Here's how the part is built. I have some questions about the finished solid (model axes, mm). A direction names the side the tool comes from. Coordinates: 2 decimals unless noted, no trailing zeros. Write each loop counter-clockwise with the first axis right and the second up, starting at its lowest first coordinate (ties: lowest second). Pieces come first, ordered by that corner, then holes.
from build123d import *

# Parameters (mm, degrees)
F0_W      = 80
F0_H      = 60
F1_DEPTH  = 10
F2_R      = 13.15
F3_DEPTH  = 10.001
F4_R      = 4
F5_DEPTH  = 10.001
F6_R      = 5
F7_W      = 14
F7_H      = 22
F8_DEPTH  = 5
F9_R      = 5
F10_R     = 13.15
F10_R_2   = 11.15
F11_DEPTH = 2.4


with BuildPart() as f1:
    # F0 (on Front) → F1 (new body)
    with BuildSketch(Plane.XZ):
        with Locations((0, 10)):
            Rectangle(F0_W, F0_H)
    extrude(amount=F1_DEPTH)

    # F2 (on face) → F3 (cut, through all)
    with BuildSketch(Plane.XZ.offset(10)):
        with Locations((0, 10)):
            Circle(F2_R)
    extrude(amount=-F3_DEPTH, mode=Mode.SUBTRACT)

    # F4 (on face) → F5 (cut, through all)
    with BuildSketch(Plane.XZ.offset(10)):
        with Locations((-31, 31)):
            Circle(F4_R)
        with Locations((31, 31)):
            Circle(F4_R)
        with Locations((-31, -11)):
            Circle(F4_R)
        with Locations((31, -11)):
            Circle(F4_R)
    extrude(amount=-F5_DEPTH, mode=Mode.SUBTRACT)

    # F6
    f6_edges = [f1.edges().sort_by_distance(p)[0] for p in [
        (40, -5, 40),
        (40, -5, -20),
        (-40, -5, -20),
        (-40, -5, 40),
    ]]
    fillet(f6_edges, radius=F6_R)

    # F7 (on face) → F8 (cut)
    with BuildSketch(Plane.XZ.offset(10)):
        Polygon((-24.5, 34.7527767497), (-31, 38.5055534995), (-37.5, 34.7527767497), (-37.5, 27.2472232503), (-31, 23.4944465005), (-24.5, 27.2472232503), align=None)
        Polygon((24.5, 34.7527767497), (24.5, 27.2472232503), (31, 23.4944465005), (37.5, 27.2472232503), (37.5, 34.7527767497), (31, 38.5055534995), align=None)
        Polygon((24.5, -7.2472232503), (24.5, -14.7527767497), (31, -18.5055534995), (37.5, -14.7527767497), (37.5, -7.2472232503), (31, -3.4944465005), align=None)
        Polygon((-24.5, -7.2472232503), (-31, -3.4944465005), (-37.5, -7.2472232503), (-37.5, -14.7527767497), (-31, -18.5055534995), (-24.5, -14.7527767497), align=None)
        with BuildLine():
            ThreePointArc((13.6106575888, 21), (16.499037969, 15.8336734651), (17.5, 10))
            ThreePointArc((17.5, 10), (16.499037969, 4.1663265349), (13.6106575888, -1))
            Line((13.6106575888, -1), (22, -1))
            Line((22, -1), (22, 21))
            Line((22, 21), (13.6106575888, 21))
        make_face()
        with BuildLine():
            ThreePointArc((-13.6106575888, 21), (0, 27.5), (13.6106575888, 21))
            Line((13.6106575888, 21), (22, 21))
            Line((22, 21), (22, 36))
            Line((22, 36), (-22, 36))
            Line((-22, 36), (-22, 21))
            Line((-22, 21), (-13.6106575888, 21))
        make_face()
        with BuildLine():
            Line((22, -1), (13.6106575888, -1))
            ThreePointArc((13.6106575888, -1), (0, -7.5), (-13.6106575888, -1))
            Line((-13.6106575888, -1), (-22, -1))
            Line((-22, -1), (-22, -16))
            Line((-22, -16), (22, -16))
            Line((22, -16), (22, -1))
        make_face()
        with BuildLine():
            ThreePointArc((-13.6106575888, -1), (-17.5, 10), (-13.6106575888, 21))
            Line((-13.6106575888, 21), (-22, 21))
            Line((-22, 21), (-22, -1))
            Line((-22, -1), (-13.6106575888, -1))
        make_face()
        with Locations((29, 10)):
            Rectangle(F7_W, F7_H)
        with Locations((-29, 10)):
            Rectangle(F7_W, F7_H)
    extrude(amount=-F8_DEPTH, mode=Mode.SUBTRACT)

    # F9
    f9_edges = [f1.edges().sort_by_distance(p)[0] for p in [
        (-22, -7.5, 21),
        (-36, -7.5, 21),
        (-22, -7.5, 36),
        (22, -7.5, 36),
        (22, -7.5, 21),
        (36, -7.5, 21),
        (-36, -7.5, -1),
        (-22, -7.5, -1),
        (-22, -7.5, -16),
        (36, -7.5, -1),
        (22, -7.5, -1),
        (22, -7.5, -16),
    ]]
    fillet(f9_edges, radius=F9_R)

    # F10 (on face) → F11 (join)
    with BuildSketch(Plane.XZ.offset(10)):
        with Locations((0, 10)):
            Circle(F10_R)
        with Locations((0, 10)):
            Circle(F10_R_2, mode=Mode.SUBTRACT)
    extrude(amount=-F11_DEPTH)


solid = f1.part
1. For pin 1 Ø5 at (x, z) = (9.5, 33) entering from -Y, with a flat end and sliding along its axis, tell me the tip position at first contact or that it passes through.
2. On a 3-axis mill with a long thin cutter (end or side, diameter ignored), from which of +Z, -Z, +X, -X, +Y, -Y can I reach the whole of each face in a straight line? I mean faces 5 (the face through (-40, -5, 10)), 6 (the face through (-13.137, -3.853, 10.578)), 7 (the face through (24.5, -8, -11)). Say none if no direction works.
3. I want a section at B-B (z = 11). List the corners of the cut face in (x, y) for me.
4. Thinking about a two-plate mould opening in X: for faces 1 (the face through (-39, -5, -18)), 2 (the face through (37.5, -8, -11)), 3 (the face through (40, -5, 10)), 4 (the face through (0, -5, 40)), which applies, pulls with the +X half, pulls with the -X half, needs draft (parallel to the pull), parting line crosses it, or undercut?
5. I want a section at D-D (x = 30). List the corners of the cut face in (y, z) for me, then the cut area to 3 significant figures.
6. I want a section at A-A (x = 0). List the corners of the cut face in (y, z) for me.
7. If I drill on line 1 (Z direction, x = 31, y = -1); line 2 (X direction, y = -7.5, z = -9); line 3 (X direction, y = -7, z = 24), over which ranges is the centre line in solid material (lowest first)?
8. I want a section at C-C (y = -6.25). State how many separate pieces and enclosed holes the cut face has, then the cut area to 3 significant figures.
Response values:
1. pin 1: stops at y = -5
2. face 5: +Z, -Z, -X, +Y, -Y
2. face 6: +Y
2. face 7: -Y
3. outline: (-40, -10) - (-36, -10) - (-36, -5) - (-17.47, -5) - (-17.47, -10) - (-11.11, -10) - (-11.11, -7.6) - (-13.11, -7.6) - (-13.11, 0) - (-40, 0) - close; (11.11, -10) - (17.47, -10) - (17.47, -5) - (36, -5) - (36, -10) - (40, -10) - (40, 0) - (13.11, 0) - (13.11, -7.6) - (11.11, -7.6) - close
4. face 1: pulls with the -X half
4. face 2: undercut
4. face 3: pulls with the +X half
4. face 4: needs draft
5. outline: (-10, -20) - (0, -20) - (0, -14.87) - (-5, -14.87) - (-5, -17.93) - (-10, -17.93) - close; (-10, -4.07) - (-5, -4.07) - (-5, -7.13) - (0, -7.13) - (0, 27.13) - (-5, 27.13) - (-5, 24.07) - (-10, 24.07) - (-10, 21) - (-5, 21) - (-5, -1) - (-10, -1) - close; (-10, 37.93) - (-5, 37.93) - (-5, 34.87) - (0, 34.87) - (0, 40) - (-10, 40) - close
5. area: 274 mm2
6. outline: (-10, -20) - (0, -20) - (0, -3.15) - (-7.6, -3.15) - (-7.6, -1.15) - (-10, -1.15) - (-10, -7.5) - (-5, -7.5) - (-5, -16) - (-10, -16) - close; (-10, 21.15) - (-7.6, 21.15) - (-7.6, 23.15) - (0, 23.15) - (0, 40) - (-10, 40) - (-10, 36) - (-5, 36) - (-5, 27.5) - (-10, 27.5) - close
7. line 1: z = -20 to -15, -7 to 27, 35 to 40
7. line 2: x = -40 to -37.5, -24.5 to -22, 22 to 24.5, 37.5 to 40
7. line 3: x = -40 to -31.88, -30.12 to -22.42, -10.5 to 10.5, 22.42 to 30.12, 31.88 to 40
8. separate pieces: 2
8. enclosed holes: 6
8. area: 1,730 mm2
